from build123d import *

# Parameters (mm, degrees)
SKETCH_1_R          = 4
SKETCH_1_R_2        = 4.1
EXTRUDE_1_DEPTH     = 15.875
FILLET_1_R          = 10
CHAMFER_1_SIZE      = 2
SKETCH_2_R          = 4.5
CUT_EXTRUDE_1_DEPTH = 20
SKETCH_3_R          = 4.5
CUT_EXTRUDE_2_DEPTH = 20


with BuildPart() as part:
    # 草图1 → 凸台-拉伸1 (new body)
    with BuildSketch(Plane.XY):
        Polygon((0, 10), (-130, 10), (-130, -20), (-110, -20), (-110, -10), (0, -10), (65, -10), (65, -30), (85, -30), (85, 10), align=None)
        Circle(SKETCH_1_R, mode=Mode.SUBTRACT)
        with Locations((-30, 0)):
            Circle(SKETCH_1_R_2, mode=Mode.SUBTRACT)
        with Locations((75, 0)):
            Circle(SKETCH_1_R_2, mode=Mode.SUBTRACT)
        with Locations((75, -20)):
            Circle(SKETCH_1_R_2, mode=Mode.SUBTRACT)
        with Locations((-120, -10)):
            Circle(SKETCH_1_R_2, mode=Mode.SUBTRACT)
    extrude(amount=EXTRUDE_1_DEPTH)

    # 圆角1
    fillet_1_edges = [part.edges().sort_by_distance(p)[0] for p in [
        (65, -10, 7.9375),
        (-110, -10, 7.9375),
    ]]
    fillet(fillet_1_edges, radius=FILLET_1_R - 0.0001)  # a hair under: the kernel refuses the full size

    # 倒角1
    chamfer_1_edges = [part.edges().sort_by_distance(p)[0] for p in [
        (-130, 10, 7.9375),
        (85, 10, 7.9375),
        (85, -30, 7.9375),
        (65, -30, 7.9375),
        (-130, -20, 7.9375),
    ]]
    chamfer(chamfer_1_edges, length=CHAMFER_1_SIZE)

    # 草图2 → 切除-拉伸1 (cut)
    with BuildSketch(Plane(origin=(0, 0, 0), x_dir=(-1, 0, 0), z_dir=(0, 0, -1))):
        with Locations((-30, 0)):
            Circle(SKETCH_2_R)
    extrude(amount=-CUT_EXTRUDE_1_DEPTH, mode=Mode.SUBTRACT)

    # 草图3 → 切除-拉伸2 (cut)
    with BuildSketch(Plane(origin=(0, 0, 0), x_dir=(-1, 0, 0), z_dir=(0, 0, -1))):
        with Locations((80, 0)):
            Circle(SKETCH_3_R)
    extrude(amount=-CUT_EXTRUDE_2_DEPTH, mode=Mode.SUBTRACT)


solid = part.part
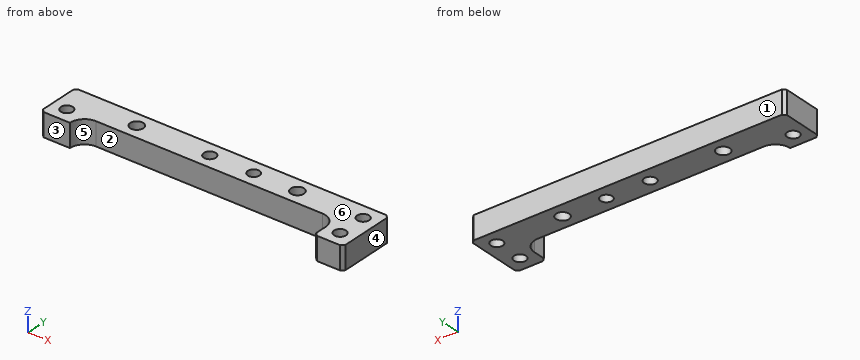
Geometry check sheet. Reference: the model listing, model coordinates, mm. Face numbers are marked on the shaded views. A direction names the side the tool comes from. Give positions to 0.01 mm unless a question says otherwise; leave off trailing zeros. Order: outer loops, then holes, each group sorted by start corner. A loop starts at its lowest first (then second) coordinate and runs counter-clockwise, first axis right, second up.
1. Sectioned sample at A-A (y = 0). Record the boundary of the cut face in (x, z) (3 decimals), then the cut area to 3 significant figures.
Completed:
outline: (-130, 0) - (-84.5, 0) - (-84.5, 15.875) - (-130, 15.875) - close; (-75.5, 0) - (-34.1, 0) - (-34.1, 15.875) - (-75.5, 15.875) - close; (-25.9, 0) - (-4, 0) - (-4, 15.875) - (-25.9, 15.875) - close; (4, 0) - (25.5, 0) - (25.5, 15.875) - (4, 15.875) - close; (34.5, 0) - (70.9, 0) - (70.9, 15.875) - (34.5, 15.875) - close; (79.1, 0) - (85, 0) - (85, 15.875) - (79.1, 15.875) - close
area: 2,740 mm2
2. Draft check along X on the marked faces 4, 5 and 6. Enter one of: pulls with the +X half, pulls with the -X half, needs draft (parallel to the pull), parting line crosses it, or undercut.
Completed:
face 4: pulls with the +X half
face 5: undercut
face 6: needs draft
3. Sectioned sample at D-D (y = -12). Record the boundary of the cut face in (x, z) (3 decimals), then the cut area to 3 significant figures.
Completed:
outline: (-130, 0) - (-123.579, 0) - (-123.579, 15.875) - (-130, 15.875) - close; (-116.421, 0) - (-106, 0) - (-106, 15.875) - (-116.421, 15.875) - close; (61, 0) - (85, 0) - (85, 15.875) - (61, 15.875) - close
area: 648 mm2
4. Scan lines: line 1 (Y direction, x = 75, z = 9.5); line 2 (X direction, y = -2, z = 9.25); line 3 (Y direction, x = -120, z = 9.5). Record each from-to range of solid material in increasing order.
Completed:
line 1: y = -30 to -24.1, -15.9 to -4.1, 4.1 to 10
line 2: x = -130 to -84.03, -75.97 to -33.58, -26.42 to -3.46, 3.46 to 25.97, 34.03 to 71.42, 78.58 to 85
line 3: y = -20 to -14.1, -5.9 to 10
5. Sectioned sample at C-C (z = 9). State how many separate pieces and enclosed holes the cut face has, then the cut area to 3 significant figures.
Completed:
separate pieces: 1
enclosed holes: 7
area: 4,540 mm2
6. Depth check by flat-ended pin: pin 1 (4 mm diameter, centred on x = -36.5, z = 4, fed in from -Y); pin 2 (4 mm diameter, centred on y = -23, z = 4.5, fed in from -X). Enter the tip coordinate at first touch or a pass-through.
Completed:
pin 1: stops at y = -10
pin 2: stops at x = 65
7. Sectioned sample at B-B (x = 30). Record the boundary of the cut face in (y, z) (3 decimals), then the cut area to 3 significant figures.
Completed:
outline: (-10, 0) - (-4.5, 0) - (-4.5, 15.875) - (-10, 15.875) - close; (4.5, 0) - (10, 0) - (10, 15.875) - (4.5, 15.875) - close
area: 175 mm2
8. Access from +Z, -Z, +X, -X, +Y, -Y to the whole of each face (thin tool, end or side, straight path). Record for the marked faces 1, 2 and 3.
Completed:
face 1: +Z, -Z, +X, -X, +Y
face 2: +Z, -Z, -Y
face 3: +Z, -Z, -X, -Y
